from build123d import *

# Parameters (mm, degrees)
SKETCH1_R             = 3.1
BOSS_EXTRUDE1_DEPTH   = 6
F_6_CLEARANCE_HOLE1_D = 3.7973


with BuildPart() as part:
    # Sketch1 → Boss-Extrude1 (new body)
    with BuildSketch(Plane(origin=(0, 0, 0), x_dir=(1, 0, 0), z_dir=(0, 1, 0))):
        with BuildLine():
            Line((-13, 15), (13, 15))
            ThreePointArc((13, 15), (14.414213562, 14.414213562), (15, 13))
            Line((15, 13), (15, -13))
            ThreePointArc((15, -13), (14.414213562, -14.414213562), (13, -15))
            Line((13, -15), (-13, -15))
            ThreePointArc((-13, -15), (-14.414213562, -14.414213562), (-15, -13))
            Line((-15, -13), (-15, 13))
            ThreePointArc((-15, 13), (-14.414213562, 14.414213562), (-13, 15))
        make_face()
        with Locations(Location((0, 0, 0), (0, 0, 270))):
            Circle(SKETCH1_R, mode=Mode.SUBTRACT)
    extrude(amount=BOSS_EXTRUDE1_DEPTH)

    # #6 Clearance Hole1 (through all)
    with Locations(Plane(origin=(0, 6, 0), x_dir=(1, 0, 0), z_dir=(0, 1, 0))):
        with Locations((-10, 10), (10, 10), (-10, -10), (10, -10)):
            Hole(F_6_CLEARANCE_HOLE1_D / 2)


solid = part.part
Here's how the part is built. I have some questions about the finished solid (model axes, mm). Give positions to 0.01 mm unless a question says otherwise; leave off trailing zeros. Loops run counter-clockwise (first coordinate to the right, second up) from the corner with the lowest first, then second, coordinate; pieces in that order, holes last. Notation, with made-up numbers: (58.5, 9.25) -> (91.5, 9.25) arc R24 ccw to (91.5, 34.25) -> close; hole circle Ø8 at (85.25, 35.5). An arc over 180 degrees is marked (long way). Answer as a JSON object with one key per item and string values. Group by question number.
Item 1: Imagine slicing it at C-C on y = 0.8. Write out the boundary of the cut face in (x, z).
Item 2: Imagine slicing it at A-A on x = 10. Write out the boundary of the cut face in (y, z), then the cut area to 3 significant figures.
Item 3: I need wall thicknesses on L1, parallel to X at y = 1.95, z = 10; L2, parallel to X at y = 4.1, z = 11.5. Which ranges of each line are inside material? Lowest first, please.
Item 4: Imagine slicing it at D-D on x = 0. Write out the boundary of the cut face in (y, z), then the cut area to 3 significant figures.
Item 5: Imagine slicing it at B-B on z = 0. Write out the boundary of the cut face in (x, y).
Item 6: Thinking about a two-plate mould opening in X: for faces 1 (the cylindrical face through (0.931, 2.958, 2.957)), 2 (the cylindrical face through (14.43, 2.96, 14.4)), 3 (the flat face through (0, 3, -15)), which applies, pulls with the +X half, pulls with the -X half, needs draft (parallel to the pull), parting line crosses it, or undercut?
Answer list:
{
 "1": {"outline": "(-15, -13) arc R2 ccw to (-13, -15) -> (13, -15) arc R2 ccw to (15, -13) -> (15, 13) arc R2 ccw to (13, 15) -> (-13, 15) arc R2 ccw to (-15, 13) -> close; hole circle Ø3.8 at (-10, -10); hole circle Ø3.8 at (-10, 10); hole circle Ø6.2 at (0, 0); hole circle Ø3.8 at (10, -10); hole circle Ø3.8 at (10, 10)"},
 "2": {"outline": "(0, -15) -> (6, -15) -> (6, -11.9) -> (0, -11.9) -> close; (0, -8.1) -> (6, -8.1) -> (6, 8.1) -> (0, 8.1) -> close; (0, 11.9) -> (6, 11.9) -> (6, 15) -> (0, 15) -> close", "area": "134 mm2"},
 "3": {"L1": "x = -15 to -11.9, -8.1 to 8.1, 11.9 to 15", "L2": "x = -15 to -11.16, -8.84 to 8.84, 11.16 to 15"},
 "4": {"outline": "(0, -15) -> (6, -15) -> (6, -3.1) -> (0, -3.1) -> close; (0, 3.1) -> (6, 3.1) -> (6, 15) -> (0, 15) -> close", "area": "143 mm2"},
 "5": {"outline": "(-15, 0) -> (-3.1, 0) -> (-3.1, 6) -> (-15, 6) -> close; (3.1, 0) -> (15, 0) -> (15, 6) -> (3.1, 6) -> close"},
 "6": {"face 1": "undercut", "face 2": "pulls with the +X half", "face 3": "needs draft"}
}
